Could you check a few things on this drawing? It's one solid part, dimensions in mm from its lowest x, y, z. A direction names the side the tool comes from. Give positions to 0.01 mm unless a question says otherwise; leave off trailing zeros. Loops run counter-clockwise (first coordinate to the right, second up) from the corner with the lowest first, then second, coordinate; pieces in that order, holes last.
Q1. Suppose I cut it at D-D (x = 12.5). List the corners of the cut face in (y, z) for me.
Q2. For the marked faces 1 and 2, which set-ups out of +Z, -Z, +X, -X, +Y, -Y let a thin tool reach every point of the face, with its end or its side?
Q3. Thinking about a two-plate mould opening in X: for the marked faces 3, 4, 5 and 6, which applies, pulls with the +X half, pulls with the -X half, needs draft (parallel to the pull), parting line crosses it, or undercut?
Q4. I need wall thicknesses on probe 1 along Z at (x, y) = (7.5, 3); probe 2 along X at (y, z) = (9.75, 7.75); probe 3 along Y at (x, z) = (13.5, 5.5). Which ranges of each line are inside material? Lowest first, please.
Q5. I'm going to push a flat-ended pin straight in: P1, Ø1.5, axis at x = 17.5, z = 7, coming from the -Y side. Where does the tip first touch, or does it pass through?
Q6. Suppose I cut it at A-A (y = 1). List the corners of the cut face in (x, z) for me, and give its area (3 significant figures).
Q7. Suppose I cut it at C-C (y = 14.25). List the corners of the cut face in (x, z) for me.
Q8. Suppose I cut it at B-B (x = 7.5). List the corners of the cut face in (y, z) for me, and give its area (4 significant figures).
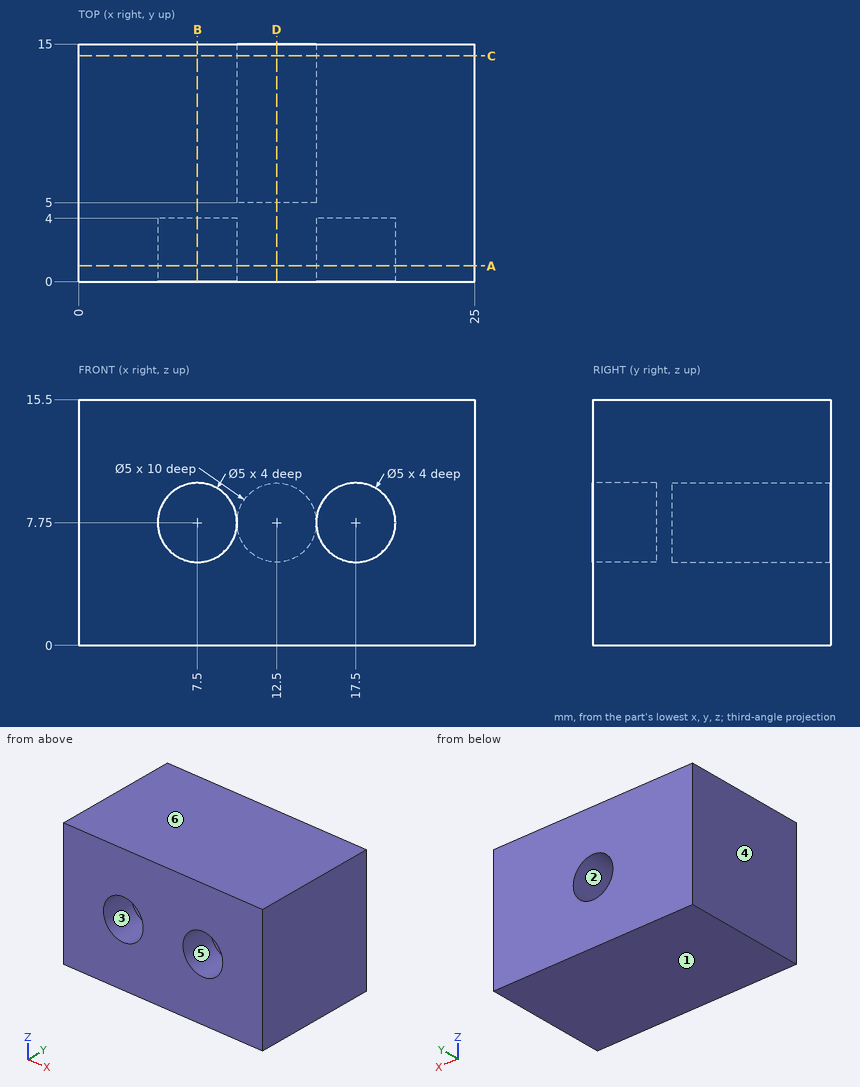
Solutions:
1. outline: (0, 0) - (15, 0) - (15, 5.25) - (5, 5.25) - (5, 10.25) - (15, 10.25) - (15, 15.5) - (0, 15.5) - close
2. face 1: -Z, +X, -X, +Y, -Y
2. face 2: +Y
3. face 3: undercut
3. face 4: pulls with the -X half
3. face 5: undercut
3. face 6: needs draft
4. probe 1: z = 0 to 5.25, 10.25 to 15.5
4. probe 2: x = 0 to 10, 15 to 25
4. probe 3: y = 0 to 5
5. P1: stops at y = 4
6. outline: (0, 0) - (25, 0) - (25, 15.5) - (0, 15.5) - close; hole circle Ø5 at (7.5, 7.75); hole circle Ø5 at (17.5, 7.75)
6. area: 348 mm2
7. outline: (0, 0) - (25, 0) - (25, 15.5) - (0, 15.5) - close; hole circle Ø5 at (12.5, 7.75)
8. outline: (0, 0) - (15, 0) - (15, 15.5) - (0, 15.5) - (0, 10.25) - (4, 10.25) - (4, 5.25) - (0, 5.25) - close
8. area: 212.5 mm2
